Job drawing, mm, ordinate dimensions from the low corner. One solid piece. Coordinates: 2 decimals unless noted, no trailing zeros. Order: outer loops, then holes, each group sorted by start corner. A loop starts at its lowest first (then second) coordinate and runs counter-clockwise, first axis right, second up. Notation, with made-up numbers: M -22.75,-38.75 L 28.25,-38.75 A10 cw 28.25,-23.75 Z; hole C 43.5,72 d3. An arc over 180 degrees is marked long. Write item = value, one per line.
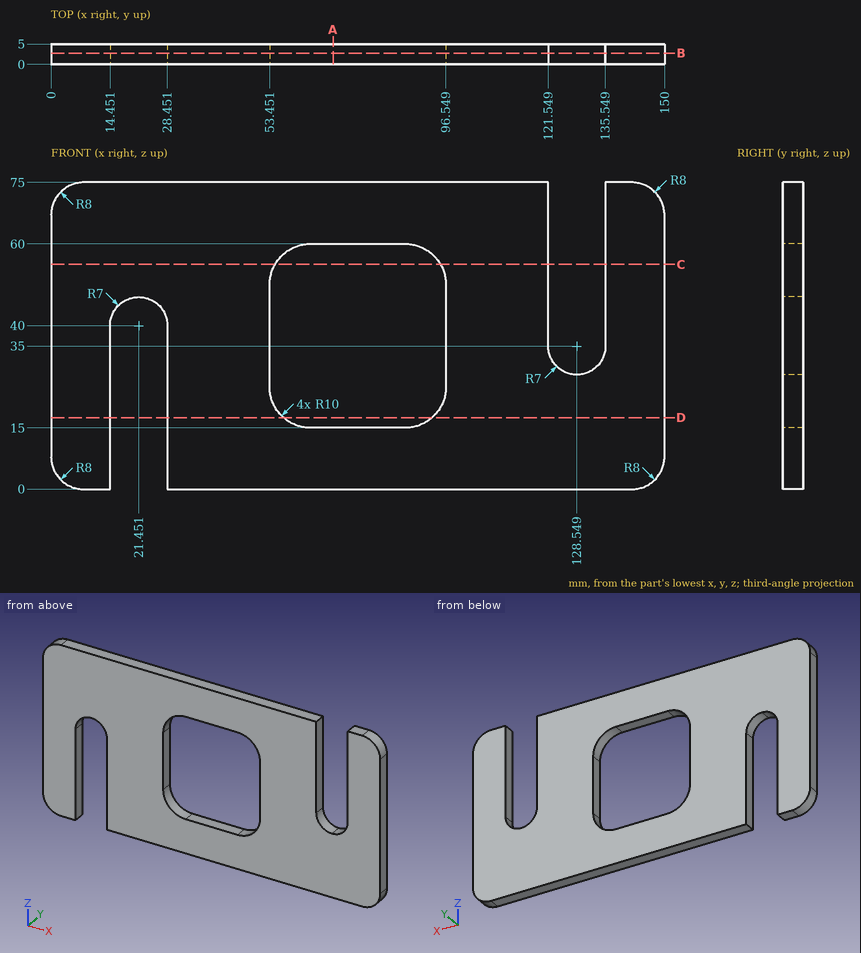
(1) Pin check, flat tip, straight feed: pin 1 Ø6 at (x, z) = (22.5, 23) entering from +Y. Stop position of the tip, or through.
Evaluation:
pin_1 = through
(2) Wall check: line 1 (X direction, y = 3.5, z = 39.5); line 2 (X direction, y = 2.6, z = 9); line 3 (Z direction, x = 84, y = 0.55). Give the ranges that are in metal, low to high. Write a range as from..to.
Evaluation:
line_1 = 0..14.45, 28.45..53.45, 96.55..121.55, 135.55..150
line_2 = 0..14.45, 28.45..150
line_3 = 0..15, 60..75
(3) Slice it at C-C, the plane z = 55. Write the cut outline in (x, y).
Evaluation:
outline = M 0,0 L 54.79,0 L 54.79,5 L 0,5 Z; M 95.21,0 L 121.55,0 L 121.55,5 L 95.21,5 Z; M 135.55,0 L 150,0 L 150,5 L 135.55,5 Z
(4) Slice it at D-D, the plane z = 17.5. Write the cut outline in (x, y), then the cut area to 3 significant figures.
Evaluation:
outline = M 0,0 L 14.45,0 L 14.45,5 L 0,5 Z; M 28.45,0 L 56.84,0 L 56.84,5 L 28.45,5 Z; M 93.16,0 L 150,0 L 150,5 L 93.16,5 Z
area = 498 mm²
(5) Slice it at B-B, the plane y = 2.75. Write the cut outline in (x, z).
Evaluation:
outline = M 0,8 A8 ccw 8,0 L 14.45,0 L 14.45,40 A7 cw 21.45,47 A7 cw 28.45,40 L 28.45,0 L 142,0 A8 ccw 150,8 L 150,67 A8 ccw 142,75 L 135.55,75 L 135.55,35 A7 cw 128.55,28 A7 cw 121.55,35 L 121.55,75 L 8,75 A8 ccw 0,67 Z; hole M 53.45,25 A10 ccw 63.45,15 L 86.55,15 A10 ccw 96.55,25 L 96.55,50 A10 ccw 86.55,60 L 63.45,60 A10 ccw 53.45,50 Z
(6) Slice it at A-A, the plane x = 69. Write the cut outline in (y, z), then the cut area to 3 significant figures.
Evaluation:
outline = M 0,0 L 5,0 L 5,15 L 0,15 Z; M 0,60 L 5,60 L 5,75 L 0,75 Z
area = 150 mm²
